from build123d import *

# Parameters (mm, degrees)
F0_R     = 25
F0_R_2   = 10.25
F1_DEPTH = 2
F2_R     = 23.25
F2_R_2   = 22
F3_DEPTH = 8
F4_SIZE  = 1
F5_R     = 1.5
F6_SIZE  = 1
F7_R     = 2


with BuildPart() as f1:
    # F0 (on Top) → F1 (new body)
    with BuildSketch(Plane.XY):
        Circle(F0_R)
        Circle(F0_R_2, mode=Mode.SUBTRACT)
    extrude(amount=F1_DEPTH)

    # F2 (on face) → F3 (join)
    with BuildSketch(Plane.XY.offset(2)):
        Circle(F2_R)
        Circle(F2_R_2, mode=Mode.SUBTRACT)
    extrude(amount=F3_DEPTH)

    # F4
    f4_edges = [f1.edges().sort_by_distance(p)[0] for p in [
        (-23.25, 0, 10),
    ]]
    chamfer(f4_edges, length=F4_SIZE)

    # F5
    f5_edges = [f1.edges().sort_by_distance(p)[0] for p in [
        (-25, 0, 0),
    ]]
    fillet(f5_edges, radius=F5_R)

    # F6
    f6_edges = [f1.edges().sort_by_distance(p)[0] for p in [
        (-10.25, 0, 0),
    ]]
    chamfer(f6_edges, length=F6_SIZE)

    # F7
    f7_edges = [f1.edges().sort_by_distance(p)[0] for p in [
        (-22, 0, 2),
    ]]
    fillet(f7_edges, radius=F7_R)


solid = f1.part
Source: CAD feature listing. Evaluate the final solid. Frame: model axes, mm. A direction names the side the tool comes from. Round coordinates to 2 decimals unless told otherwise and drop trailing zeros. Loops run counter-clockwise (first coordinate to the right, second up) from the corner with the lowest first, then second, coordinate; pieces in that order, holes last. Notation, with made-up numbers: (-9.5, 44.25) -> (13.5, 44.25) arc R9 ccw to (13.5, 50.25) -> close; hole circle Ø6 at (74.25, 50). An arc over 180 degrees is marked (long way). Answer as a JSON object with one key per item and string values. Group by question number.
Q1. Access query for faces 4 (the flat face through (17, -17, 2)), 5 (the cylindrical face through (23.846, 7.509, 1.746)). Directions: +Z, -Z, +X, -X, +Y, -Y. A direction counts if a zero-diameter tool reaches every point of the face in a straight line with its end or side. Return the directions, or none.
Q2. Section query D-D (z = 2.75). Output: boundary loops of the cut face in (x, y), plus the area to 3 significant figures.
Q3. Contact query for flat-ended pins moving along their axis: P1, Ø1, axis at y = -7, z = 8.5, coming from the -X side; P2, Ø5, axis at x = -6.5, y = -8, coming from the +Z side; P3, Ø18.5, axis at x = 0, y = 0, coming from the -Z side; P4, Ø1.5, axis at y = 1, z = 7.5, coming from the +X side. Output: stop coordinate, or through.
Q4. Section query C-C (z = 7.5). Output: boundary loops of the cut face in (x, y), plus the area to 3 significant figures.
Q5. Ray query, line 1 (Y direction, x = 0, z = 7); line 2 (Y direction, x = 0, z = 1.6); line 3 (Z direction, x = -10, y = 6.5). Return the intervals inside material, ascending. Write a range as from..to.
Q6. Mould query, pull axis Y, two halves, no side actions, for faces 1 (the cylindrical face through (-4.769, -21.477, 6.958)), 2 (the cylindrical face through (22.176, 6.984, 5.451)), 3 (the flat face through (10, 6, 0)). Classes: pulls with the +Y half, pulls with the -Y half, needs draft (parallel to the pull), parting line crosses it, or undercut.
Q7. Section query A-A (y = 0). Output: boundary loops of the cut face in (x, z).
Completed:
{
 "1": {"face 4": "+Z", "face 5": "+Z, -Z"},
 "2": {"outline": "circle Ø46.5 at (0, 0); hole circle Ø43.12 at (0, 0)", "area": "238 mm²"},
 "3": {"P1": "x = -22.32", "P2": "z = 2", "P3": "through", "P4": "x = 23.25"},
 "4": {"outline": "circle Ø46.5 at (0, 0); hole circle Ø44 at (0, 0)", "area": "178 mm²"},
 "5": {"line 1": "-23.25..-22, 22..23.25", "line 2": "-25..-10.25, 10.25..25", "line 3": "0..2"},
 "6": {"face 1": "undercut", "face 2": "parting line crosses it", "face 3": "needs draft"},
 "7": {"outline": "(-25, 1.5) arc R1.5 ccw to (-23.5, 0) -> (-11.25, 0) -> (-10.25, 1) -> (-10.25, 2) -> (-20, 2) arc R2 cw to (-22, 4) -> (-22, 10) -> (-22.25, 10) -> (-23.25, 9) -> (-23.25, 2) -> (-25, 2) -> close; (10.25, 1) -> (11.25, 0) -> (23.5, 0) arc R1.5 ccw to (25, 1.5) -> (25, 2) -> (23.25, 2) -> (23.25, 9) -> (22.25, 10) -> (22, 10) -> (22, 4) arc R2 cw to (20, 2) -> (10.25, 2) -> close"}
}
